Read the model definition and answer for the solid it produces. Units are mm, in the model's axes. A direction names the side the tool comes from. Coordinates: 2 decimals unless noted, no trailing zeros. Write each loop counter-clockwise with the first axis right and the second up, starting at its lowest first coordinate (ties: lowest second). Pieces come first, ordered by that corner, then holes.
(1) Determine the mould class of faces 3 (the cylindrical face through (9.7, -0.6, 3.2)), 4 (the flat face through (7.198, 2.745, 3.24)), 5 (the flat face through (2, -2, 0)) for opening direction X: pulls with the +X half, pulls with the -X half, needs draft (parallel to the pull), parting line crosses it, or undercut.
(2) Which of the six approach directions +Z, -Z, +X, -X, +Y, -Y give full straight-line access (tool end or side, diameter ignored) to faces 1 (the flat face through (0, 0, 2.5)), 2 (the flat face through (4, 0, 4))?
(3) The part is cut by section D-D, the plane x = 5.5. Determine the outline of the cut face in (y, z).
(4) Given pin 1 (4 mm diameter, centred on x = 9.5, y = 2, fed in from -Z); pin 2 (1 mm diameter, centred on x = 6.5, z = 1, fed in from -Y), each flat-ended and moving along its own axis, determine where each tip first touches the part or whether it passes through.
(5) The part is cut by section C-C, the plane x = 13.5. Determine the outline of the cut face in (y, z), and give its area (3 significant figures).
(6) The part is cut by section B-B, the plane x = 10.5. Determine the outline of the cut face in (y, z), and give its area (3 significant figures).
(7) The part is cut by section A-A, the plane z = 2.9. Determine the outline of the cut face in (x, y) (3 decimals), and give its area (3 significant figures).
(8) Straight lines are drawn through the part: line 1 along Z through (x, y) = (4, 2); line 2 along X through (y, z) = (1.25, 1.7); line 3 along Y through (x, z) = (10.5, 3.1). For each, find the intervals that lie inside material, in ascending order.
```python
from build123d import *

# Parameters (mm, degrees)
SKETCH_R     = 3.5
PAD_DEPTH    = 2.5
SKETCH001_R  = 1
PAD001_DEPTH = 1.5


with BuildPart() as part:
    # Sketch → Pad (new body)
    with BuildSketch(Plane.XY):
        Circle(SKETCH_R)
        Polygon((0.331619, 2.200149), (0.766363, 2.484489), (0.965391, 2.004656), (1.464632, 2.148221), (1.513384, 1.63104), (2.032762, 1.621073), (1.926907, 1.1125), (2.420272, 0.949887), (2.169215, 0.495109), (2.59273, 0.194298), (2.218778, -0.166274), (2.534813, -0.578554), (2.071194, -0.812884), (2.251666, -1.3), (1.739575, -1.387265), (1.768449, -1.905935), (1.253387, -1.838381), (1.128098, -2.342519), (0.65583, -2.126149), (0.38751, -2.57096), (0, -2.225), (-0.38751, -2.57096), (-0.65583, -2.126149), (-1.128098, -2.342519), (-1.253387, -1.838381), (-1.768449, -1.905935), (-1.739575, -1.387265), (-2.251666, -1.3), (-2.071194, -0.812884), (-2.534813, -0.578554), (-2.218778, -0.166274), (-2.59273, 0.194298), (-2.169215, 0.495109), (-2.420272, 0.949887), (-1.926907, 1.1125), (-2.032762, 1.621073), (-1.513384, 1.63104), (-1.464632, 2.148221), (-0.965391, 2.004656), (-0.766363, 2.484489), (-0.331619, 2.200149), (0, 2.6), align=None, mode=Mode.SUBTRACT)
    extrude(amount=PAD_DEPTH)

    # Sketch001 (on Face45 of Pad) → Pad001 (join)
    with BuildSketch(Plane.XY.offset(2.5)):
        with BuildLine():
            ThreePointArc((0.375, 3.479853), (-3.5, 0), (0.375, -3.479853))
            Line((0.375, -3.479853), (14.214286, -1.988487))
            ThreePointArc((14.214286, -1.988487), (16, 0), (14.214286, 1.988487))
            Line((0.375, 3.479853), (14.214286, 1.988487))
        make_face()
        with Locations((10.5, 0)):
            Circle(SKETCH001_R, mode=Mode.SUBTRACT)
    extrude(amount=PAD001_DEPTH)


solid = part.part
```
Computed:
1. face 3: undercut
1. face 4: pulls with the +X half
1. face 5: needs draft
2. face 1: -Z
2. face 2: +Z, +X, -X, +Y, -Y
3. outline: (-2.93, 2.5) - (2.93, 2.5) - (2.93, 4) - (-2.93, 4) - close
4. pin 1: stops at z = 2.5
4. pin 2: passes through
5. outline: (-2.07, 2.5) - (2.07, 2.5) - (2.07, 4) - (-2.07, 4) - close
5. area: 6.20 mm2
6. outline: (-2.39, 2.5) - (-1, 2.5) - (-1, 4) - (-2.39, 4) - close; (1, 2.5) - (2.39, 2.5) - (2.39, 4) - (1, 4) - close
6. area: 4.17 mm2
7. outline: (0.375, -3.48) - (14.214, -1.988) arc R2 ccw to (14.214, 1.988) - (0.375, 3.48) arc R3.5 ccw (long way) to start; hole circle Ø2 at (10.5, 0)
7. area: 99.8 mm2
8. line 1: z = 2.5 to 4
8. line 2: x = -3.27 to -1.96, 1.96 to 3.27
8. line 3: y = -2.39 to -1, 1 to 2.39
